For this review, take the finished solid that the model builds, in its own axes (mm). Face numbers are marked on the shaded views. A direction names the side the tool comes from. Give positions to 0.01 mm unless a question says otherwise; leave off trailing zeros. Write each loop counter-clockwise with the first axis right and the second up, starting at its lowest first coordinate (ties: lowest second). Pieces come first, ordered by that corner, then holes.
1) We need section B-B on x = 0. Give the boundary of the cut face in (y, z).
2) We need section C-C on z = -20.5. Give the boundary of the cut face in (x, y) (3 decimals), and give its area (3 significant figures).
3) We need section D-D on x = -27.5. Give the boundary of the cut face in (y, z), and give its area (3 significant figures).
4) For P1, Ø15, axis at x = 0, y = 0, coming from the -Z side; P2, Ø7.5, axis at x = 14, z = -24, coming from the +Y side; P3, Ø1, axis at x = -38, y = 18, coming from the -Z side; P4, Ø5, axis at x = 11, z = -29.5, coming from the +Y side, all flat-tipped, find the tip position at first contact; note any pin that passes through.
5) We need section A-A on y = 0. Give the boundary of the cut face in (x, z), and give its area (3 significant figures).
6) Machinability: for the marked faces 5, 6, 7 and 8, which of the approach directions +Z, -Z, +X, -X, +Y, -Y give a long, thin tool a straight path to every point of the face, cutting with its end or side? Answer none if there is none.
7) Draft analysis for pull direction Y (two halves, no side actions). For the marked faces 1, 2, 3 and 4, state which applies: pulls with the +Y half, pulls with the -Y half, needs draft (parallel to the pull), parting line crosses it, or undercut.
8) Wall thickness on line 1 along Z through (x, y) = (2, -16); line 2 along Z through (x, y) = (31.5, 30.5); line 3 along X through (y, z) = (-4, -6): over which ranges is each line inside the solid? List them lowest first.
from build123d import *

# Parameters (mm, degrees)
F1_DEPTH = 12.7
F0_R     = 2.9972
F0_R_2   = 20.574
F2_DEPTH = 9.652
F3_DEPTH = 9.652
F4_DEPTH = 38.1


with BuildPart() as f1:
    # F0 (on Top) → F1 (new body)
    with BuildSketch(Plane.XY):
        with BuildLine():
            Line((-24.1480973609, 6.4704631866), (-48.2961947219, 12.9409263732))
            ThreePointArc((-48.2961947219, 12.9409263732), (-49.9999, 0), (-48.2961947219, -12.9409263732))
            Line((-48.2961947219, -12.9409263732), (-24.1480973609, -6.4704631866))
            ThreePointArc((-24.1480973609, -6.4704631866), (-24.99995, 0), (-24.1480973609, 6.4704631866))
        make_face()
    extrude(amount=F1_DEPTH)



with BuildPart() as f1b:
    # F0 (on Top) → F1, piece 2 (new body)
    with BuildSketch(Plane.XY):
        with BuildLine():
            Line((17.6776341743, 17.6776341743), (35.3552683486, 35.3552683486))
            ThreePointArc((35.3552683486, 35.3552683486), (24.99995, 43.3011835867), (12.9409263732, 48.2961947219))
            Line((12.9409263732, 48.2961947219), (6.4704631866, 24.1480973609))
            ThreePointArc((6.4704631866, 24.1480973609), (12.499975, 21.6505917933), (17.6776341743, 17.6776341743))
        make_face()
    extrude(amount=F1_DEPTH)


with BuildPart() as f1c:
    # F0 (on Top) → F1, piece 3 (new body)
    with BuildSketch(Plane.XY):
        with BuildLine():
            ThreePointArc((12.9409263732, -48.2961947219), (24.99995, -43.3011835867), (35.3552683486, -35.3552683486))
            Line((35.3552683486, -35.3552683486), (17.6776341743, -17.6776341743))
            ThreePointArc((17.6776341743, -17.6776341743), (12.499975, -21.6505917933), (6.4704631866, -24.1480973609))
            Line((6.4704631866, -24.1480973609), (12.9409263732, -48.2961947219))
        make_face()
    extrude(amount=F1_DEPTH)


with BuildPart() as f1_1:
    add(f1.part)

    add(f1b.part)  # F2 merges F1b

    add(f1c.part)  # F2 merges F1c
    # F0 (on Top) → F2 (join)
    with BuildSketch(Plane.XY):
        with BuildLine():
            ThreePointArc((35.3552683486, -35.3552683486), (46.1938842376, -19.1341333499), (49.9999, 0))
            ThreePointArc((49.9999, 0), (46.1938842376, 19.1341333499), (35.3552683486, 35.3552683486))
            Line((35.3552683486, 35.3552683486), (17.6776341743, 17.6776341743))
            ThreePointArc((17.6776341743, 17.6776341743), (12.499975, 21.6505917933), (6.4704631866, 24.1480973609))
            Line((6.4704631866, 24.1480973609), (12.9409263732, 48.2961947219))
            ThreePointArc((12.9409263732, 48.2961947219), (-24.99995, 43.3011835867), (-48.2961947219, 12.9409263732))
            Line((-48.2961947219, 12.9409263732), (-24.1480973609, 6.4704631866))
            ThreePointArc((-24.1480973609, 6.4704631866), (-24.99995, 0), (-24.1480973609, -6.4704631866))
            Line((-24.1480973609, -6.4704631866), (-48.2961947219, -12.9409263732))
            ThreePointArc((-48.2961947219, -12.9409263732), (-24.99995, -43.3011835867), (12.9409263732, -48.2961947219))
            Line((12.9409263732, -48.2961947219), (6.4704631866, -24.1480973609))
            ThreePointArc((6.4704631866, -24.1480973609), (12.499975, -21.6505917933), (17.6776341743, -17.6776341743))
            Line((17.6776341743, -17.6776341743), (35.3552683486, -35.3552683486))
        make_face()
        with Locations((-15.0495, -26.0664986285)):
            Circle(F0_R, mode=Mode.SUBTRACT)
        with Locations((-15.0495, 26.0664986285)):
            Circle(F0_R, mode=Mode.SUBTRACT)
        Circle(F0_R_2, mode=Mode.SUBTRACT)
        with Locations((30.099, 0)):
            Circle(F0_R, mode=Mode.SUBTRACT)
        Circle(F0_R_2)
        with BuildLine():
            ThreePointArc((12.2967221242, -3.175), (-12.7, 0), (12.2967221242, 3.175))
            Line((12.2967221242, 3.175), (19.05, 3.175))
            Line((19.05, 3.175), (19.05, 0))
            Line((19.05, 0), (19.05, -3.175))
            Line((19.05, -3.175), (12.2967221242, -3.175))
        make_face(mode=Mode.SUBTRACT)
    extrude(amount=-F2_DEPTH)

    # F3 (add): faces of the model
    f3_faces = [f1_1.faces().sort_by_distance(p)[0] for p in [
        (-38.4460981424, 0, 0),
        (19.2230490712, 33.2952976677, 0),
        (19.2230490712, -33.2952976677, 0),
    ]]
    extrude(f3_faces, amount=F3_DEPTH)

    # F0 (on Top) → F4 (join)
    with BuildSketch(Plane.XY):
        Circle(F0_R_2)
        with BuildLine():
            ThreePointArc((12.2967221242, -3.175), (-12.7, 0), (12.2967221242, 3.175))
            Line((12.2967221242, 3.175), (19.05, 3.175))
            Line((19.05, 3.175), (19.05, 0))
            Line((19.05, 0), (19.05, -3.175))
            Line((19.05, -3.175), (12.2967221242, -3.175))
        make_face(mode=Mode.SUBTRACT)
    extrude(amount=-F4_DEPTH)


solid = f1_1.part
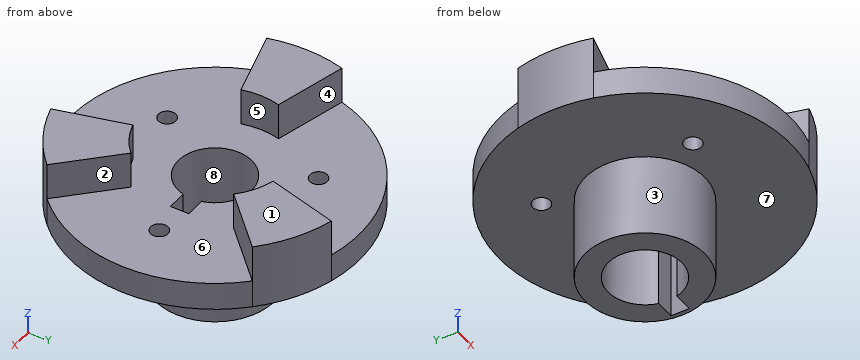
Results list:
1. outline: (-50, -9.65) - (-20.57, -9.65) - (-20.57, -38.1) - (-12.7, -38.1) - (-12.7, 0) - (-50, 0) - close; (12.7, -38.1) - (20.57, -38.1) - (20.57, -9.65) - (50, -9.65) - (50, 0) - (12.7, 0) - close
2. outline: circle Ø41.148 at (0, 0); hole (12.297, -3.175) - (19.05, -3.175) - (19.05, 3.175) - (12.297, 3.175) arc R12.7 ccw (long way) to start
2. area: 782 mm2
3. outline: (-41.76, -9.65) - (41.76, -9.65) - (41.76, 0) - (7.37, 0) - (7.37, 12.7) - (-7.37, 12.7) - (-7.37, 0) - (-41.76, 0) - close
3. area: 993 mm2
4. P1: passes through
4. P2: stops at y = 17.84
4. P3: stops at z = -9.65
4. P4: stops at y = 18.74
5. outline: (-50, -9.65) - (-20.57, -9.65) - (-20.57, -38.1) - (-12.7, -38.1) - (-12.7, 0) - (-25, 0) - (-25, 12.7) - (-50, 12.7) - close; (19.05, -38.1) - (20.57, -38.1) - (20.57, -9.65) - (27.1, -9.65) - (27.1, 0) - (19.05, 0) - close; (33.1, -9.65) - (50, -9.65) - (50, 0) - (33.1, 0) - close
5. area: 1,190 mm2
6. face 5: +Z, +X
6. face 6: +Z
6. face 7: -Z
6. face 8: +Z, -Z
7. face 1: needs draft
7. face 2: undercut
7. face 3: parting line crosses it
7. face 4: pulls with the +Y half
8. line 1: z = -38.1 to 0
8. line 2: z = -9.65 to 0
8. line 3: x = -49.84 to -12.05, 12.05 to 49.84
